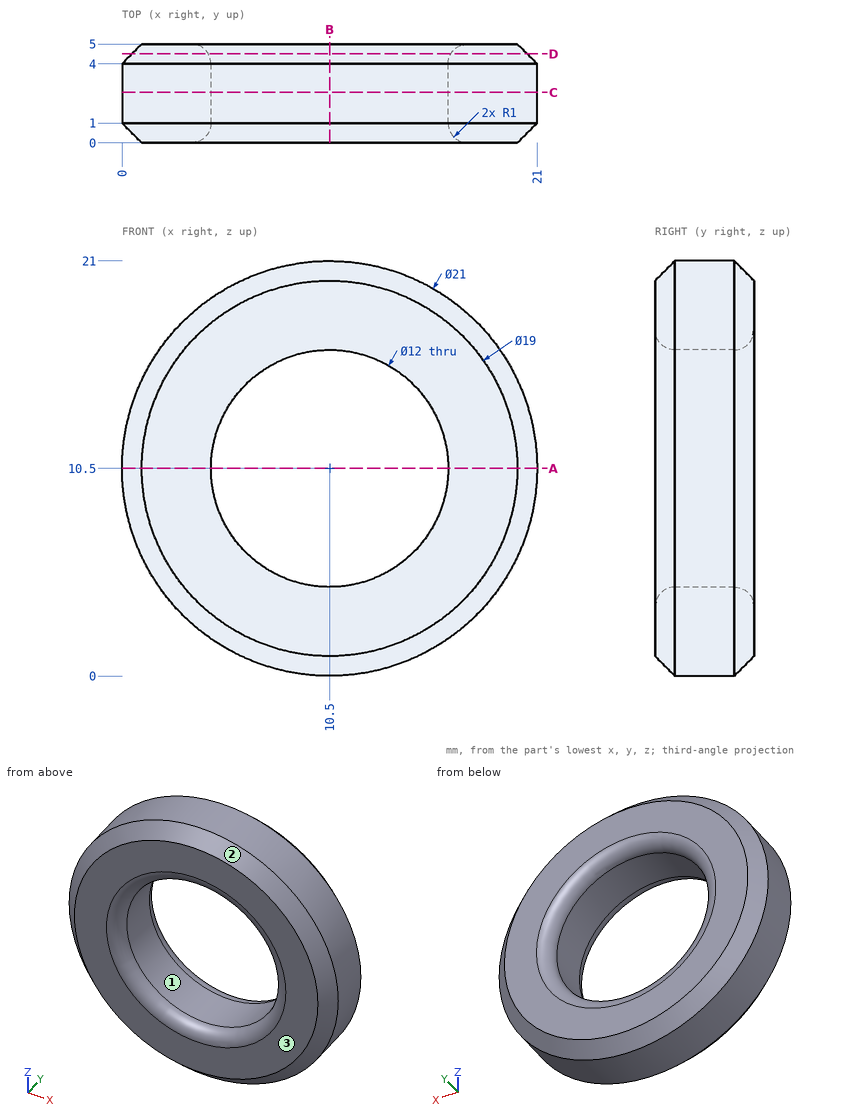
Design review of the part shown in the three views and the two pictorial views. Dimensions are in mm from the part's minimum x, y and z. Round coordinates to 2 decimals unless told otherwise and drop trailing zeros. Loops run counter-clockwise (first coordinate to the right, second up) from the corner with the lowest first, then second, coordinate; pieces in that order, holes last.
(1) Wall thickness on line 1 along Z through (x, y) = (10.5, 1.75); line 2 along Z through (x, y) = (12, 1.1): over which ranges is each line inside the solid? List them lowest first.
Returned:
line 1: z = 0 to 4.5, 16.5 to 21
line 2: z = 0.11 to 4.69, 16.31 to 20.89
(2) Mouldability with a two-part tool opening along Z and no side actions: class the marked faces 1, 2 and 3 as released by +Z, released by -Z, zero draft, split by the parting line, or undercut.
Returned:
face 1: undercut
face 2: split by the parting line
face 3: zero draft
(3) We need section B-B (x = 10.5). Give the boundary of the cut face in (y, z).
Returned:
outline: (0, 1) - (1, 0) - (4, 0) - (5, 1) - (5, 3.5) arc R1 ccw to (4, 4.5) - (1, 4.5) arc R1 ccw to (0, 3.5) - close; (0, 17.5) arc R1 ccw to (1, 16.5) - (4, 16.5) arc R1 ccw to (5, 17.5) - (5, 20) - (4, 21) - (1, 21) - (0, 20) - close
(4) Clearance check with a flat-ended pin moving along its axis: P1, Ø1, axis at y = 2, z = 13, coming from the +X side. State where the tip first meets the part, or that it passes through.
Returned:
P1: stops at x = 20.81
(5) We need section A-A (z = 10.5). Give the boundary of the cut face in (x, y).
Returned:
outline: (0, 1) - (1, 0) - (3.5, 0) arc R1 ccw to (4.5, 1) - (4.5, 4) arc R1 ccw to (3.5, 5) - (1, 5) - (0, 4) - close; (16.5, 1) arc R1 ccw to (17.5, 0) - (20, 0) - (21, 1) - (21, 4) - (20, 5) - (17.5, 5) arc R1 ccw to (16.5, 4) - close
(6) We need section D-D (y = 4.5). Give the boundary of the cut face in (x, z), plus the area to 3 significant figures.
Returned:
outline: circle Ø20 at (10.5, 10.5); hole circle Ø12.27 at (10.5, 10.5)
area: 196 mm2
(7) We need section C-C (y = 2.55). Give the boundary of the cut face in (x, z), plus the area to 3 significant figures.
Returned:
outline: circle Ø21 at (10.5, 10.5); hole circle Ø12 at (10.5, 10.5)
area: 233 mm2
